from build123d import *

# Parameters (mm, degrees)
SKETCH1_R           = 5
BOSS_EXTRUDE1_DEPTH = 12.5
SKETCH2_W           = 7.5
SKETCH2_H           = 40
BOSS_EXTRUDE4_DEPTH = 5
SKETCH4_R           = 2.5
CUT_EXTRUDE1_DEPTH  = 100
FILLET1_R           = 2.5
FILLET2_R           = 2.5


with BuildPart() as part:
    # Sketch1 → Boss-Extrude1 (new body)
    with BuildSketch(Plane(origin=(0, 0, 0), x_dir=(1, 0, 0), z_dir=(0, 1, 0))):
        with Locations(Location((0.037460471, 3.715413796, 0), (0, 0, 270))):
            Circle(SKETCH1_R)
        with BuildLine():
            ThreePointArc((-1.612539529, 1.667390359), (0.037460471, 1.085413796), (1.687460471, 1.667390359))
            Line((1.687460471, 1.667390359), (1.687460471, 5.76407365))
            ThreePointArc((1.687460471, 5.76407365), (0.037460471, 6.346050212), (-1.612539529, 5.76407365))
            Line((-1.612539529, 5.76407365), (-1.612539529, 1.667390359))
        make_face(mode=Mode.SUBTRACT)
    extrude(amount=BOSS_EXTRUDE1_DEPTH)

    # Sketch2 → Boss-Extrude4 (add)
    with BuildSketch(Plane(origin=(0, 12.5, 0), x_dir=(1, 0, 0), z_dir=(0, 1, 0))):
        Polygon((4.77657028, 5.309414491), (1.02657028, -1.185776038), (35.667586431, -21.185776038), (39.417586431, -14.690585509), align=None)
        with Locations((0.037460471, 27.022602935)):
            Rectangle(SKETCH2_W, SKETCH2_H)
        Polygon((-4.701649339, 5.309414491), (-0.951649339, -1.185776038), (-35.59266549, -21.185776038), (-39.34266549, -14.690585509), align=None)
    extrude(amount=-BOSS_EXTRUDE4_DEPTH)

    # Sketch4 → Cut-Extrude1 (cut)
    with BuildSketch(Plane(origin=(0, 12.5, 0), x_dir=(1, 0, 0), z_dir=(0, 1, 0))):
        with Locations(Location((0.037460471, 16.216050212, 0), (0, 0, 270))):
            Circle(SKETCH4_R)
        with Locations(Location((0.037460471, 28.716050212, 0), (0, 0, 270))):
            Circle(SKETCH4_R)
        with Locations(Location((0.037460471, 41.216050212, 0), (0, 0, 270))):
            Circle(SKETCH4_R)
        with Locations(Location((-10.788016154, -2.533674249, 0), (0, 0, 270))):
            Circle(SKETCH4_R)
        with Locations(Location((-21.613492779, -8.78339871, 0), (0, 0, 270))):
            Circle(SKETCH4_R)
        with Locations(Location((-32.438969404, -15.033123172, 0), (0, 0, 270))):
            Circle(SKETCH4_R)
        with Locations(Location((10.862937095, -2.533674249, 0), (0, 0, 90))):
            Circle(SKETCH4_R)
        with Locations(Location((21.68841372, -8.78339871, 0), (0, 0, 90))):
            Circle(SKETCH4_R)
        with Locations(Location((32.513890345, -15.033123172, 0), (0, 0, 90))):
            Circle(SKETCH4_R)
    extrude(amount=-CUT_EXTRUDE1_DEPTH, mode=Mode.SUBTRACT)

    # Fillet1
    fillet1_edges = [part.edges().sort_by_distance(p)[0] for p in [
        (4.77657028, 10, -5.309414491),
        (1.02657028, 10, 1.185776038),
        (-3.712539529, 10, -7.022602935),
        (3.787460471, 10, -7.022602935),
        (-4.701649339, 10, -5.309414491),
        (-0.951649339, 10, 1.185776038),
    ]]
    fillet(fillet1_edges, radius=FILLET1_R)

    # Fillet2
    fillet2_edges = [part.edges().sort_by_distance(p)[0] for p in [
        (39.417586431, 10, 14.690585509),
        (35.667586431, 10, 21.185776038),
        (-3.712539529, 10, -47.022602935),
        (3.787460471, 10, -47.022602935),
        (-39.34266549, 10, 14.690585509),
        (-35.59266549, 10, 21.185776038),
    ]]
    fillet(fillet2_edges, radius=FILLET2_R)


solid = part.part
Design review of the part built by this model. Coordinates are the model's own, in mm. A direction names the side the tool comes from. Give positions to 0.01 mm unless a question says otherwise; leave off trailing zeros. Write each loop counter-clockwise with the first axis right and the second up, starting at its lowest first coordinate (ties: lowest second). Pieces come first, ordered by that corner, then holes. Notation, with made-up numbers: M 62.5,-16 L 71.5,-16 A21 cw 71.5,3 Z; hole C 38.25,41.25 d11. An arc over 180 degrees is marked long. Return JSON: item names as keys, results as strings. Group by question number.
Item 1: The part is to be moulded in two halves that separate along X. For faces 1 (the flat face through (21.6, 10.035, 4.404)), 2 (the cylindrical face through (-0.9, 10, -26.4)), 3 (the flat face through (-37.46, 10.04, 17.95)), say which applies: pulls with the +X half, pulls with the -X half, needs draft (parallel to the pull), parting line crosses it, or undercut.
Item 2: Tool access review of faces 4 (the flat face through (-17.33, 10.04, 10.64)), 5 (the flat face through (-3.713, 10, -26)), 6 (the cylindrical face through (0.012, 6.162, -1.086)): name each direction out of +Z, -Z, +X, -X, +Y, -Y from which nothing blocks a thin tool from reaching the whole face with its end or side.
Item 3: Wall thickness on line 1 along X through (y, z) = (8.5, 16); line 2 along Z through (x, y) = (0, 5.5); line 3 along Y through (x, z) = (11.5, 5.5): over which ranges is each line inside the solid? List them lowest first.
Item 4: Clearance check with flat-ended pins moving along their axes: pin 1 Ø6.5 at (x, z) = (1, -36.5) entering from -Y; pin 2 Ø5.5 at (y, z) = (10.5, -28.5) entering from +X; pin 3 Ø3 at (x, z) = (-32.44, 15.03) entering from -Y; pin 4 Ø4.5 at (y, z) = (8, -2.5) entering from +X. State where each tip first meets the part, or that it passes through.
Item 5: Take a section at B-B (z = -29.5). Give the boundary of the cut face in (x, y).
Item 6: Take a section at D-D (y = 5). Give the boundary of the cut face in (x, z), plus the area to 3 significant figures.
Item 7: Take a section at A-A (z = 4). Give the boundary of the cut face in (x, y).
Item 8: Take a section at C-C (x = 31). Give the boundary of the cut face in (y, z).
Return value:
{
 "1": {"face 1": "pulls with the +X half", "face 2": "undercut", "face 3": "pulls with the -X half"},
 "2": {"face 4": "+Z, +Y, -Y", "face 5": "-Z, -X, +Y, -Y", "face 6": "+Y, -Y"},
 "3": {"line 1": "x = -38.4 to -34.74, -30.13 to -26.61, 26.69 to 30.21, 34.82 to 38.47", "line 2": "z = -8.72 to -6.35, -1.09 to 1.28", "line 3": "y = 7.5 to 12.5"},
 "4": {"pin 1": "stops at y = 7.5", "pin 2": "stops at x = 3.79", "pin 3": "passes through", "pin 4": "stops at x = 13.54"},
 "5": {"outline": "M -3.71,7.5 L -2.34,7.5 L -2.34,12.5 L -3.71,12.5 Z; M 2.41,7.5 L 3.79,7.5 L 3.79,12.5 L 2.41,12.5 Z"},
 "6": {"outline": "C 0.04,-3.72 d10; hole M -1.61,-5.76 A2.63 ccw 1.69,-5.76 L 1.69,-1.67 A2.63 ccw -1.61,-1.67 Z", "area": "62.4 mm2"},
 "7": {"outline": "M -20.83,7.5 L -12.81,7.5 L -12.81,12.5 L -20.83,12.5 Z; M -8.76,7.5 L -5.83,7.5 L -5.83,12.5 L -8.76,12.5 Z; M 5.9,7.5 L 8.84,7.5 L 8.84,12.5 L 5.9,12.5 Z; M 12.89,7.5 L 20.9,7.5 L 20.9,12.5 L 12.89,12.5 Z"},
 "8": {"outline": "M 7.5,9.83 L 12.5,9.83 L 12.5,13.04 L 7.5,13.04 Z; M 7.5,17.02 L 12.5,17.02 L 12.5,18.49 L 7.5,18.49 Z"}
}
